Verification items for the finished model (mm, model axes). A direction names the side the tool comes from. Give positions to 0.01 mm unless a question says otherwise; leave off trailing zeros. Loops run counter-clockwise (first coordinate to the right, second up) from the corner with the lowest first, then second, coordinate; pieces in that order, holes last. Notation, with made-up numbers: (46.25, 10.5) - (88.25, 10.5) arc R28 ccw to (88.25, 35.5) - close; hole circle Ø4 at (43, 80). An arc over 180 degrees is marked (long way). Answer in a Markdown table with one row per item.
```python
from build123d import *
from build123d.topology import SkipClean

# Parameters (mm, degrees)
BOSS_EXTRUDE1_DEPTH = 9.525
BOSS_EXTRUDE2_START = 50.8
SKETCH2_R           = 4.7625
BOSS_EXTRUDE2_DEPTH = 50.8


with BuildPart() as part:
    # Sketch1 → Boss-Extrude1 (new body)
    with BuildSketch(Plane.XY):
        with BuildLine():
            Line((-2.54, 4.028623369), (-2.54, 0))
            Line((-2.54, 0), (2.54, 0))
            Line((2.54, 0), (2.54, 4.028623369))
            ThreePointArc((2.54, 4.028623369), (0, 4.7625), (-2.54, 4.028623369))
        make_face()
        with BuildLine():
            Line((2.54, 0), (-2.54, 0))
            Line((-2.54, 0), (-2.54, 4.028623369))
            ThreePointArc((-2.54, 4.028623369), (-2.300506058, -4.170021358), (4.7625, 0))
            ThreePointArc((4.7625, 0), (4.170021358, 2.300506058), (2.54, 4.028623369))
            Line((2.54, 4.028623369), (2.54, 0))
        make_face()
        with BuildLine():
            Line((-2.54, 10.16), (-2.54, 4.028623369))
            ThreePointArc((-2.54, 4.028623369), (0, 4.7625), (2.54, 4.028623369))
            Line((2.54, 4.028623369), (2.54, 10.16))
            Line((2.54, 10.16), (-2.54, 10.16))
        make_face()
    extrude(amount=BOSS_EXTRUDE1_DEPTH)

    # Sketch2 → Boss-Extrude2 (add)
    with SkipClean():  # the faces are left unmerged after this step: merging them gives an invalid solid
        with BuildSketch(Plane(origin=(0, 0, 0), x_dir=(-1, 0, 0), z_dir=(0, 0, -1)).offset(BOSS_EXTRUDE2_START)):
            Circle(SKETCH2_R)
        extrude(amount=-BOSS_EXTRUDE2_DEPTH)


solid = part.part
```
Q1. Sectioned sample at D-D (y = 8). Record the cut outline in (x, z) (3 decimals).
Completed:
| item | result |
|---|---|
| outline | (-2.54, 0) - (2.54, 0) - (2.54, 9.525) - (-2.54, 9.525) - close |
Q2. Tool access check on faces 1 (the face through (0, 0, -50.8)), 2 (the face through (-2.54, 7, 5)), 3 (the face through (2.54, 7, 5)). Record the directions out of +Z, -Z, +X, -X, +Y, -Y that give a thin tool (end or side, any length) a straight path to the whole face; none if there is none.
Completed:
| item | result |
|---|---|
| face 1 | -Z, +X, -X, +Y, -Y |
| face 2 | +Z, -Z, -X, +Y |
| face 3 | +Z, -Z, +X, +Y |
Q3. Sectioned sample at A-A (x = 0). Record the cut outline in (y, z) (1 decimal).
Completed:
| item | result |
|---|---|
| outline | (-4.8, -50.8) - (4.8, -50.8) - (4.8, 0) - (10.2, 0) - (10.2, 9.5) - (-4.8, 9.5) - close |
Q4. Go/stop test with flat-tipped pins: P1, Ø1.5, axis at x = 0.5, y = 7, coming from the -Z side; P2, Ø1.8, axis at y = 6.5, z = 6, coming from the +X side; P3, Ø1.8, axis at y = 8, z = 2.5, coming from the -X side. Record where each tip stops, or that it passes through.
Completed:
| item | result |
|---|---|
| P1 | z = 0 |
| P2 | x = 2.54 |
| P3 | x = -2.54 |
Q5. Sectioned sample at C-C (y = 2). Record the cut outline in (x, z) (3 decimals), and give its area (3 significant figures).
Completed:
| item | result |
|---|---|
| outline | (-4.322, -50.8) - (4.322, -50.8) - (4.322, 9.525) - (-4.322, 9.525) - close |
| area | 521 mm^2 |
Q6. Sectioned sample at B-B (z = -17.5). Record the cut outline in (x, y) (1 decimal), and give its area (3 significant figures).
Completed:
| item | result |
|---|---|
| outline | circle Ø9.5 at (0, 0) |
| area | 71.3 mm^2 |
Q7. Thickness scan on line 1 (X direction, y = 6.75, z = 6); line 2 (Z direction, x = -1.5, y = 5.75) (3 decimals); line 3 (Y direction, x = -3.25, z = -41.5). Record the ranges inside material, lowest first.
Completed:
| item | result |
|---|---|
| line 1 | -2.54 to 2.54 |
| line 2 | 0 to 9.525 |
| line 3 | -3.48 to 3.48 |
